For this review, use the dimensioned drawing (mm, ordinates from the lowest corner) and the shaded views. A direction names the side the tool comes from. Coordinates: 2 decimals unless noted, no trailing zeros. Loops run counter-clockwise (first coordinate to the right, second up) from the corner with the lowest first, then second, coordinate; pieces in that order, holes last.
1. Clearance check with flat-ended pins moving along their axes: P1, Ø2, axis at x = 3, y = 10, coming from the +Z side; P2, Ø1.5, axis at y = 11, z = 3, coming from the -X side; P3, Ø2, axis at x = 14.5, z = 2, coming from the +Y side. State where each tip first meets the part, or that it passes through.
2. Take a section at C-C, the plane z = 0.5. State the section outline as (x, y) points.
3. Mouldability with a two-part tool opening along X and no side actions: class the marked faces 3, 4 and 5 as pulls with the +X half, pulls with the -X half, needs draft (parallel to the pull), parting line crosses it, or undercut.
4. Take a section at A-A, the plane y = 10. State the section outline as (x, z) points, then the cut area to 3 significant figures.
5. To check wall thickness, follow probe 1 along Y at (x, z) = (10, 0.8); probe 2 along Y at (x, z) = (10.5, 1.5). State the ranges of each line that lie inside material, in increasing order.
6. Machinability: for the marked faces 1 and 2, which of the approach directions +Z, -Z, +X, -X, +Y, -Y give a long, thin tool a straight path to every point of the face, cutting with its end or side? Answer none if there is none.
7. Take a section at D-D, the plane y = 4. State the section outline as (x, z) points.
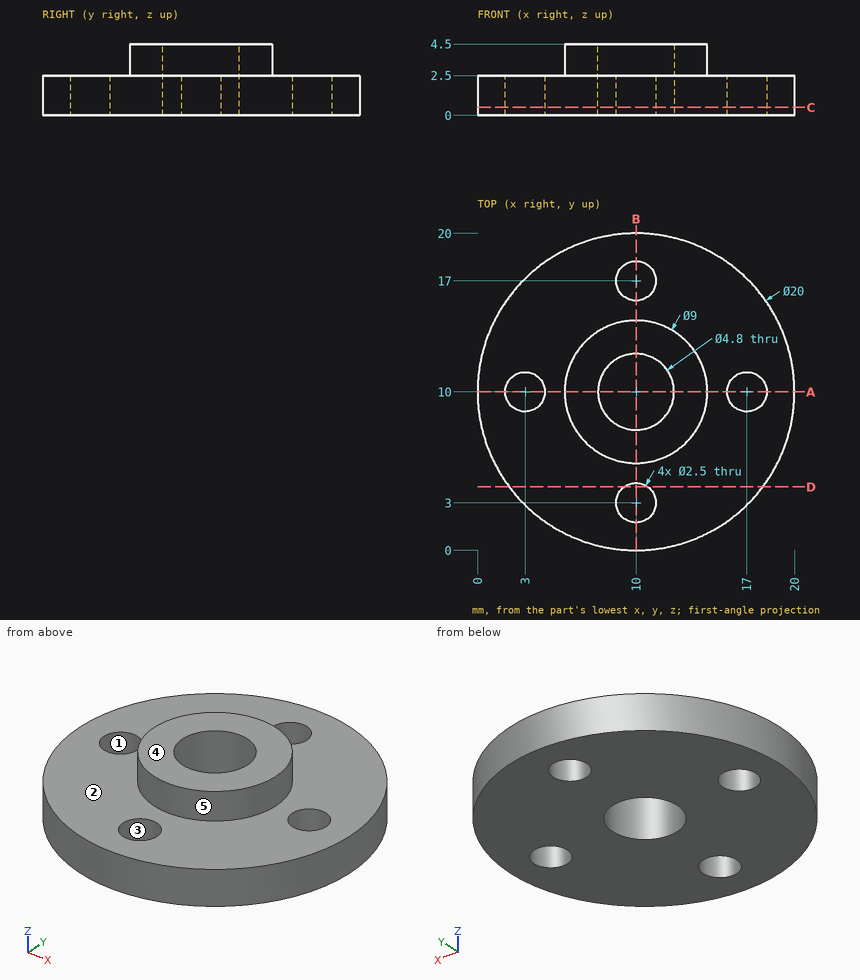
Results list:
1. P1: passes through
1. P2: stops at x = 0.01
1. P3: stops at y = 19.37
2. outline: circle Ø20 at (10, 10); hole circle Ø2.5 at (3, 10); hole circle Ø4.8 at (10, 10); hole circle Ø2.5 at (10, 3); hole circle Ø2.5 at (10, 17); hole circle Ø2.5 at (17, 10)
3. face 3: undercut
3. face 4: needs draft
3. face 5: parting line crosses it
4. outline: (0, 0) - (1.75, 0) - (1.75, 2.5) - (0, 2.5) - close; (4.25, 0) - (7.6, 0) - (7.6, 4.5) - (5.5, 4.5) - (5.5, 2.5) - (4.25, 2.5) - close; (12.4, 0) - (15.75, 0) - (15.75, 2.5) - (14.5, 2.5) - (14.5, 4.5) - (12.4, 4.5) - close; (18.25, 0) - (20, 0) - (20, 2.5) - (18.25, 2.5) - close
4. area: 33.9 mm2
5. probe 1: y = 0 to 1.75, 4.25 to 7.6, 12.4 to 15.75, 18.25 to 20
5. probe 2: y = 0.01 to 1.85, 4.15 to 7.65, 12.35 to 15.85, 18.15 to 19.99
6. face 1: +Z, -Z
6. face 2: +Z
7. outline: (2, 0) - (9.25, 0) - (9.25, 2.5) - (2, 2.5) - close; (10.75, 0) - (18, 0) - (18, 2.5) - (10.75, 2.5) - close
